```python
from build123d import *

# Parameters (mm, degrees)
F0_R         = 1.5
F0_W         = 2.1
F0_H         = 6.2
F1_DEPTH     = 2
F2_R         = 3
F4_DEPTH     = 2.001
F5_R         = 5
F6_T1_DEPTH  = 16.7901994578
F7_W         = 7
F7_H         = 16
F7_R         = 3.25
F8_DEPTH     = 2.001
F9_R         = 5
F10_T1_DEPTH = 2


# Not quite as in the source:
# - a fillet or chamfer that OpenCascade refuses, or shapes differently, is made with other operations: its cross-section is extruded or revolved along the edge and cut away or added


with BuildPart() as f1:
    # F0 (on Top) → F1 (new body)
    with BuildSketch(Plane.XY):
        Polygon((-13, -32), (13, -32), (13, 32), (7.5, 32), (7.5, 22), (-7.5, 22), (-7.5, 32), (-13, 32), align=None)
        with Locations((0, -29)):
            Circle(F0_R, mode=Mode.SUBTRACT)
        with Locations((-10.55, 19)):
            Circle(F0_R, mode=Mode.SUBTRACT)
        with Locations((-10.55, 27)):
            Rectangle(F0_W, F0_H, mode=Mode.SUBTRACT)
        with Locations((10.55, 19)):
            Circle(F0_R, mode=Mode.SUBTRACT)
        with Locations((10.55, 27)):
            Rectangle(F0_W, F0_H, mode=Mode.SUBTRACT)
    extrude(amount=F1_DEPTH)

    # F2
    f2_edges = [f1.edges().sort_by_distance(p)[0] for p in [
        (13, 32, 1),
        (7.5, 22, 1),
        (-7.5, 22, 1),
        (-13, 32, 1),
    ]]
    fillet(f2_edges, radius=F2_R)

    # F3 (on face) → F4 (cut, through all)
    with BuildSketch(Plane.XY.offset(2)):
        Polygon((-9.65, -28.1011469207), (-13, -3), (-13, -33), (13, -33), (13, -3), (9.65, -28.1011469207), (0, -32), align=None)
    extrude(amount=-F4_DEPTH, mode=Mode.SUBTRACT)

    # F5
    f5_edges = [f1.edges().sort_by_distance(p)[0] for p in [
        (9.65, -28.101147, 1),
        (-9.65, -28.101147, 1),
        (13, -3, 1),
        (0, -32, 1),
        (-13, -3, 1),
    ]]
    fillet(f5_edges, radius=F5_R)

    # F6: fillet of radius 3 on 2 edges, made by hand

    # F6_s2 → F6_t1 (cut)
    with BuildSketch(Plane.XY.offset(-7.3950997289)):
        with BuildLine():
            ThreePointArc((-7.5, 29.0419601084), (-8.2087121525, 30.9784517816), (-10, 32))
            Line((-10, 32), (-7.5, 32))
            Line((-7.5, 32), (-7.5, 29.0419601084))
        make_face()
        with BuildLine():
            ThreePointArc((10, 32), (8.2087121525, 30.9784517816), (7.5, 29.0419601084))
            Line((7.5, 29.0419601084), (7.5, 32))
            Line((7.5, 32), (10, 32))
        make_face()
    extrude(amount=F6_T1_DEPTH, mode=Mode.SUBTRACT)

    # F7 (on face) → F8 (cut, through all)
    with BuildSketch(Plane.XY.offset(2)):
        Polygon((10, 14), (0, 18), (-10, 14), (-10, 2), (10, 2), align=None)
        Polygon((-5.5, -2), (-10, -2), (-6.8708787487, -25.4461290331), (-5.5, -26), align=None)
        Polygon((6.8708787487, -25.4461290331), (10, -2), (5.5, -2), (5.5, -26), align=None)
        with Locations((0, -10)):
            Rectangle(F7_W, F7_H)
        with Locations((0, -23)):
            Circle(F7_R)
    extrude(amount=-F8_DEPTH, mode=Mode.SUBTRACT)

    # F9
    f9_edges = [f1.edges().sort_by_distance(p)[0] for p in [
        (-10, 14, 1),
        (0, 18, 1),
        (10, 14, 1),
        (-10, 2, 1),
        (10, 2, 1),
    ]]
    fillet(f9_edges, radius=F9_R)

    # F10: fillet of radius 1 on 12 edges, made by hand

    # F10_s2 → F10_t1 (join)
    with BuildSketch(Plane.XY):
        with BuildLine():
            ThreePointArc((-8.8576734794, -2), (-9.6100985971, -2.3413222015), (-9.8488849195, -3.1322871156))
            Line((-9.8488849195, -3.1322871156), (-10, -2))
            Line((-10, -2), (-8.8576734794, -2))
        make_face()
        with BuildLine():
            ThreePointArc((-3.5, -3), (-3.2071067812, -2.2928932188), (-2.5, -2))
            Line((-2.5, -2), (-3.5, -2))
            Line((-3.5, -2), (-3.5, -3))
        make_face()
        with BuildLine():
            ThreePointArc((6.5, -2), (5.7928932188, -2.2928932188), (5.5, -3))
            Line((5.5, -3), (5.5, -2))
            Line((5.5, -2), (6.5, -2))
        make_face()
        with BuildLine():
            ThreePointArc((-5.5, -3), (-5.7928932188, -2.2928932188), (-6.5, -2))
            Line((-6.5, -2), (-5.5, -2))
            Line((-5.5, -2), (-5.5, -3))
        make_face()
        with BuildLine():
            ThreePointArc((3.5, -3), (3.2071067812, -2.2928932188), (2.5, -2))
            Line((2.5, -2), (3.5, -2))
            Line((3.5, -2), (3.5, -3))
        make_face()
        with BuildLine():
            ThreePointArc((9.8488849195, -3.1322871156), (9.6100985971, -2.3413222015), (8.8576734794, -2))
            Line((8.8576734794, -2), (10, -2))
            Line((10, -2), (9.8488849195, -3.1322871156))
        make_face()
        with BuildLine():
            ThreePointArc((-3.5, -17), (-3.2071067812, -17.7071067812), (-2.5, -18))
            Line((-2.5, -18), (-3.5, -18))
            Line((-3.5, -18), (-3.5, -17))
        make_face()
        with BuildLine():
            ThreePointArc((2.5, -18), (3.2071067812, -17.7071067812), (3.5, -17))
            Line((3.5, -17), (3.5, -18))
            Line((3.5, -18), (2.5, -18))
        make_face()
        with BuildLine():
            ThreePointArc((-6.3312640971, -25.6641475042), (-6.7468030166, -25.3498829497), (-6.9478689438, -24.8692507652))
            Line((-6.9478689438, -24.8692507652), (-6.8708787487, -25.4461290331))
            Line((-6.8708787487, -25.4461290331), (-6.3312640971, -25.6641475042))
        make_face()
        with BuildLine():
            ThreePointArc((6.9478689438, -24.8692507652), (6.7468030166, -25.3498829497), (6.3312640971, -25.6641475042))
            Line((6.3312640971, -25.6641475042), (6.8708787487, -25.4461290331))
            Line((6.8708787487, -25.4461290331), (6.9478689438, -24.8692507652))
        make_face()
        with BuildLine():
            ThreePointArc((5.5, -24.5174390315), (5.9408070965, -25.346476604), (6.8746065934, -25.4446228861))
            Line((6.8746065934, -25.4446228861), (5.5, -26))
            Line((5.5, -26), (5.5, -24.5174390315))
        make_face()
        with BuildLine():
            ThreePointArc((-6.8746065934, -25.4446228861), (-5.9408070965, -25.346476604), (-5.5, -24.5174390315))
            Line((-5.5, -24.5174390315), (-5.5, -26))
            Line((-5.5, -26), (-6.8746065934, -25.4446228861))
        make_face()
    extrude(amount=F10_T1_DEPTH)


solid = f1.part
```
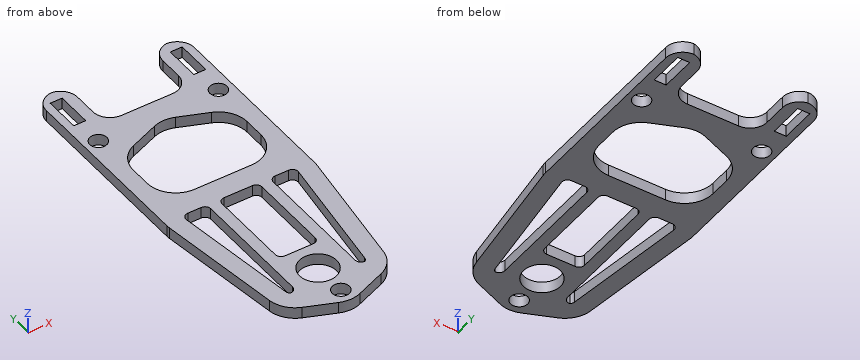
Here's how the part is built. I have some questions about the finished solid (model axes, mm). Coordinates: 2 decimals unless noted, no trailing zeros. Order: outer loops, then holes, each group sorted by start corner. A loop starts at its lowest first (then second) coordinate and runs counter-clockwise, first axis right, second up. Notation, with made-up numbers: (5, -35) - (56, -35) arc R25 ccw to (56, -16) - close; hole circle Ø3 at (40.25, -1). An arc over 180 degrees is marked (long way). One line per question, with ' | ' between items. Start each with the question number.
1. If we section it at B-B (x = 0): Write out the boundary of the cut face in (y, z), and give its area (3 significant figures).
2. I'm going to push flat-ended pins straight in: pin 1 Ø1 at (y, z) = (-18.5, 0.5) entering from +X; pin 2 Ø0.6 at (x, z) = (-1, 1) entering from +Y; pin 3 Ø0.6 at (y, z) = (-15, 1.5) entering from -X. Where does each tip first touch, or does it pass through?
3. If we section it at D-D (z = 1.3): Give the number of separate pieces and of enclosed holes in the cut face, and give its area (3 significant figures).
4. If we section it at C-C (y = -23): Write out the boundary of the cut face in (x, z).
5. Please list where these lines run through material, in increasing order: line 1 along X through (y, z) = (25.5, 1.4); line 2 along X through (y, z) = (-20, 1.45); line 3 along X through (y, z) = (22.5, 1.2). Write a range as [from, to].
6. If we section it at A-A (y = 19): Write out the boundary of the cut face in (x, z).
Model answer:
1) outline: (-31.61, 0) - (-30.5, 0) - (-30.5, 2) - (-31.61, 2) - close; (-27.5, 0) - (-26.25, 0) - (-26.25, 2) - (-27.5, 2) - close; (-19.75, 0) - (-18, 0) - (-18, 2) - (-19.75, 2) - close; (-2, 0) - (2, 0) - (2, 2) - (-2, 2) - close; (17.61, 0) - (22, 0) - (22, 2) - (17.61, 2) - close | area: 25.0 mm²
2) pin 1: stops at x = 11 | pin 2: stops at y = 22 | pin 3: stops at x = -11.44
3) separate pieces: 1 | enclosed holes: 10 | area: 767 mm²
4) outline: (-10.33, 0) - (-7.2, 0) - (-7.2, 2) - (-10.33, 2) - close; (-5.5, 0) - (-3.25, 0) - (-3.25, 2) - (-5.5, 2) - close; (3.25, 0) - (5.5, 0) - (5.5, 2) - (3.25, 2) - close; (7.2, 0) - (10.33, 0) - (10.33, 2) - (7.2, 2) - close
5) line 1: x = [-13, -11.6], [-9.5, -7.5], [7.5, 9.5], [11.6, 13] | line 2: x = [-10.73, -7.6], [-5.5, -1.25], [1.25, 5.5], [7.6, 10.73] | line 3: x = [-13, -6.16], [6.16, 13]
6) outline: (-13, 0) - (-12.05, 0) - (-12.05, 2) - (-13, 2) - close; (-9.05, 0) - (9.05, 0) - (9.05, 2) - (-9.05, 2) - close; (12.05, 0) - (13, 0) - (13, 2) - (12.05, 2) - close
